The figure shows three views and two pictorial views of one solid part (mm, origin at its lowest corner). Answer the questions. A direction names the side the tool comes from. Coordinates: 2 decimals unless noted, no trailing zeros. Write each loop counter-clockwise with the first axis right and the second up, starting at its lowest first coordinate (ties: lowest second). Pieces come first, ordered by that corner, then holes.
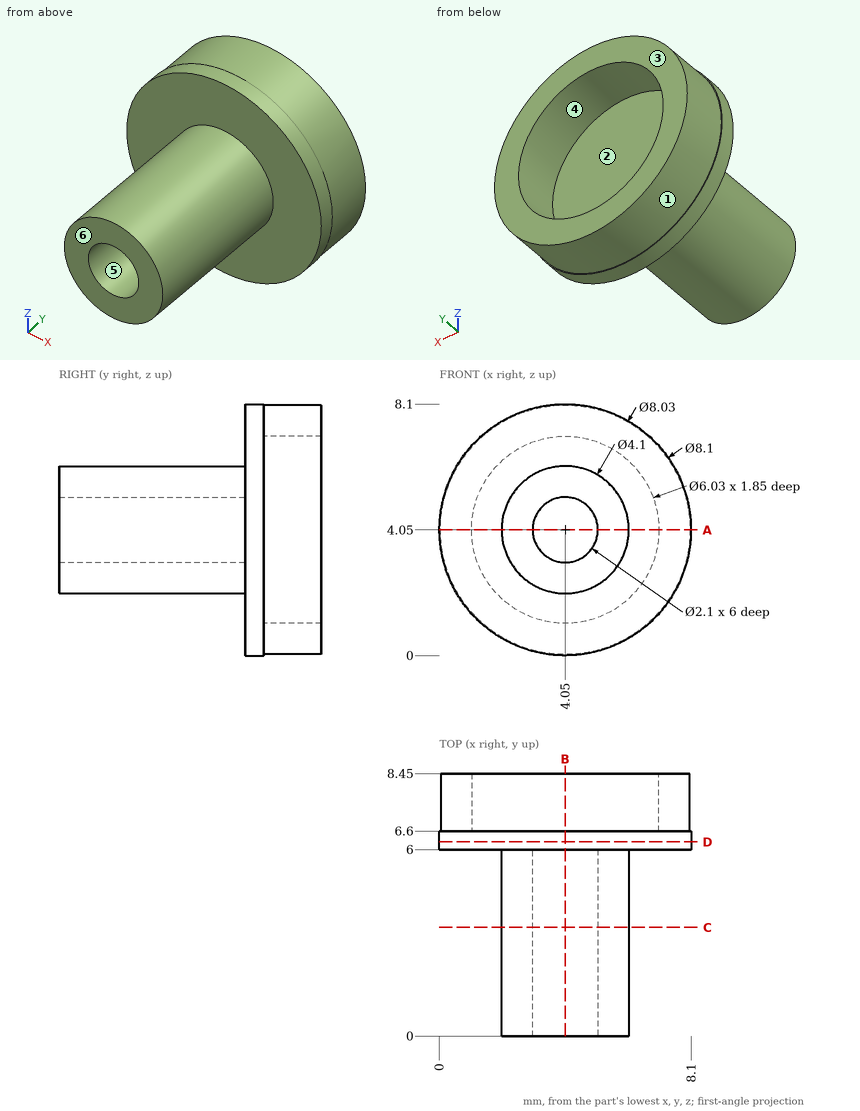
Q1. Given pin 1 (3 mm diameter, centred on x = 4.5, y = 5.5, fed in from -Z); pin 2 (3.5 mm diameter, centred on x = 4.05, z = 4.05, fed in from +Y); pin 3 (2 mm diameter, centred on x = 2, y = 1.5, fed in from -Z); pin 4 (2 mm diameter, centred on y = 4.5, z = 4.5, fed in from -X), each flat-ended and moving along its own axis, determine where each tip first touches the part or whether it passes through.
Answers below:
pin 1: stops at z = 0
pin 2: stops at y = 6.6
pin 3: stops at z = 2.29
pin 4: stops at x = 2
Q2. Determine the mould class of the marked faces 1, 2 and 3 for opening direction X: released by +X, released by -X, zero draft, split by the parting line, or undercut.
Answers below:
face 1: split by the parting line
face 2: undercut
face 3: zero draft
Q3. The part is cut by section B-B, the plane x = 4.05. Write down the section's boundary in (y, z) (3 decimals), then the cut area to 3 significant figures.
Answers below:
outline: (0, 2) - (6, 2) - (6, 0) - (6.6, 0) - (6.6, 0.035) - (8.45, 0.035) - (8.45, 1.035) - (6.6, 1.035) - (6.6, 7.065) - (8.45, 7.065) - (8.45, 8.065) - (6.6, 8.065) - (6.6, 8.1) - (6, 8.1) - (6, 6.1) - (0, 6.1) - (0, 5.1) - (6, 5.1) - (6, 3) - (0, 3) - close
area: 20.6 mm2
Q4. Find the intervals of material crossed by probe 1 along Z at (x, y) = (4.05, 2.5); probe 2 along X at (y, z) = (7.95, 4.05) (3 decimals), in increasing order.
Answers below:
probe 1: z = 2 to 3, 5.1 to 6.1
probe 2: x = 0.035 to 1.035, 7.065 to 8.065
Q5. The part is cut by section A-A, the plane z = 4.05. Write down the section's boundary in (x, y) (3 decimals).
Answers below:
outline: (0, 6) - (2, 6) - (2, 0) - (3, 0) - (3, 6) - (5.1, 6) - (5.1, 0) - (6.1, 0) - (6.1, 6) - (8.1, 6) - (8.1, 6.6) - (8.065, 6.6) - (8.065, 8.45) - (7.065, 8.45) - (7.065, 6.6) - (1.035, 6.6) - (1.035, 8.45) - (0.035, 8.45) - (0.035, 6.6) - (0, 6.6) - close
Q6. The part is cut by section C-C, the plane y = 3.5. Write down the section's boundary in (x, z), then the cut area to 3 significant figures.
Answers below:
outline: circle Ø4.1 at (4.05, 4.05); hole circle Ø2.1 at (4.05, 4.05)
area: 9.74 mm2
Q7. Which of the six approach directions +Z, -Z, +X, -X, +Y, -Y give full straight-line access (tool end or side, diameter ignored) to the marked faces 4, 5 and 6?
Answers below:
face 4: +Y
face 5: -Y
face 6: +Z, -Z, +X, -X, -Y
Q8. The part is cut by section D-D, the plane y = 6.25. Write down the section's boundary in (x, z).
Answers below:
outline: circle Ø8.1 at (4.05, 4.05)
